The listing builds one solid part. Answer for the finished solid, in the listing's coordinates (mm). A direction names the side the tool comes from. Give positions to 0.01 mm unless a question says otherwise; leave off trailing zeros. Order: outer loops, then holes, each group sorted by start corner. A loop starts at its lowest first (then second) coordinate and runs counter-clockwise, first axis right, second up.
```python
from build123d import *

# Parameters (mm, degrees)
SKETCH2_W           = 30
SKETCH2_H           = 30
BOSS_EXTRUDE1_DEPTH = 15
SKETCH3_R           = 2.5
CUT_EXTRUDE1_DEPTH  = 5


with BuildPart() as part:
    # Sketch2 → Boss-Extrude1 (new body, symmetric)
    with BuildSketch(Plane(origin=(0, 0, 0), x_dir=(0, 0, -1), z_dir=(1, 0, 0))):
        with Locations((15, 15)):
            Rectangle(SKETCH2_W, SKETCH2_H)
    extrude(amount=BOSS_EXTRUDE1_DEPTH, both=True)

    # Sketch3 → Cut-Extrude1 (cut, symmetric)
    with BuildSketch(Plane.XY):
        with Locations((0, 15)):
            Circle(SKETCH3_R)
    extrude(amount=CUT_EXTRUDE1_DEPTH, both=True, mode=Mode.SUBTRACT)


solid = part.part
```
1) Given P1, Ø4, axis at x = 12, z = -4, coming from the -Y side, flat-ended and moving along its own axis, determine where the tip first touches the part or whether it passes through.
Geometry says:
P1: stops at y = 0
2) Find section A-A (z = -4.5). Write down the section's boundary in (x, y).
Geometry says:
outline: (-15, 0) - (15, 0) - (15, 30) - (-15, 30) - close; hole circle Ø5 at (0, 15)
3) Find section B-B (x = 0). Write down the section's boundary in (y, z).
Geometry says:
outline: (0, -30) - (30, -30) - (30, 0) - (17.5, 0) - (17.5, -5) - (12.5, -5) - (12.5, 0) - (0, 0) - close
4) Straight lines are drawn through the part: probe 1 along Y at (x, z) = (0, -3.5); probe 2 along X at (y, z) = (12.75, -1.5). For each, find the intervals that lie inside material, in ascending order.
Geometry says:
probe 1: y = 0 to 12.5, 17.5 to 30
probe 2: x = -15 to -1.09, 1.09 to 15
5) A tool of negligible diameter and unlimited length cuts with its end or side. For faces 1 (the flat face through (0, 15, -5)), 2 (the flat face through (0, 15, -30)), from which of +Z, -Z, +X, -X, +Y, -Y can it reach the whole face along a straight path? Write none if from no direction.
Geometry says:
face 1: +Z
face 2: -Z, +X, -X, +Y, -Y
6) Find section C-C (y = 15). Write down the section's boundary in (x, z), then the cut area to 3 significant figures.
Geometry says:
outline: (-15, -30) - (15, -30) - (15, 0) - (2.5, 0) - (2.5, -5) - (-2.5, -5) - (-2.5, 0) - (-15, 0) - close
area: 875 mm2
7) For a pull along Y with two mould halves and no side action, classify faces 3 (the flat face through (0, 30, -15)), 4 (the flat face through (0, 0, -15)), 5 (the cylindrical face through (-0.54, 12.56, -2.46)) as +Y half, -Y half, draft (parallel to the pull), parting line (faces both ways), or undercut.
Geometry says:
face 3: +Y half
face 4: -Y half
face 5: undercut
